Geometry: final body of the model. Coordinates: model frame, mm. Face numbers are marked on the shaded views. A direction names the side the tool comes from. Coordinates: 2 decimals unless noted, no trailing zeros. Loops run counter-clockwise (first coordinate to the right, second up) from the corner with the lowest first, then second, coordinate; pieces in that order, holes last. Notation, with made-up numbers: (5.5, 20.5) - (25.5, 20.5) arc R24 ccw to (25.5, 51.5) - close; hole circle Ø11 at (12, 54.25). An arc over 180 degrees is marked (long way). Put each result on its own line as item: value. Start each with the question number.
1) Material intervals for line 1 along X through (y, z) = (2.2, 0); line 2 along X through (y, z) = (9.5, 0); line 3 along Y through (x, z) = (-10.5, -5), sorted ascending. Write a range as from..to.
2) Section C-C on x = 5. Output: boundary loops of the cut face in (y, z), and give its area (3 significant figures).
3) Contact query for flat-ended pins moving along their axis: pin 1 Ø6 at (x, z) = (-10, 0) entering from -Y; pin 2 Ø1.5 at (x, z) = (-3, -2) entering from +Y; pin 3 Ø1 at (x, y) = (12.5, 10.5) entering from -Z. Output: stop coordinate, or through.
4) Reachability of the marked faces 3, 4 and 5 from +Z, -Z, +X, -X, +Y, -Y: full face, straight path, thin tool, end or side. Return the list, or none.
5) Section B-B on x = 8.5. Output: boundary loops of the cut face in (y, z).
6) Draft query along X for the marked faces 1 and 2. Return one class per face: +X half, -X half, draft (parallel to the pull), parting line (faces both ways), or undercut.
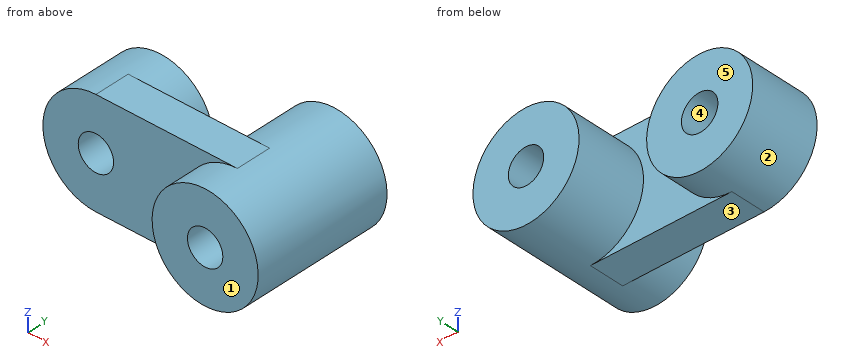
```python
from build123d import *

# Parameters (mm, degrees)
CROQUIS1_R                   = 2.5
SALIENTE_EXTRUIR1_DEPTH      = 5
CROQUIS2_R                   = 7.5
CROQUIS2_R_2                 = 2.58081611
SALIENTE_EXTRUIR2_DEPTH      = 5
SALIENTE_EXTRUIR3_DEPTH      = 10
SALIENTE_EXTRUIR3_DEPTH_BACK = 10
CROQUIS3_R                   = 7.5
CROQUIS3_R_2                 = 2.5


with BuildPart() as part:
    # Croquis1 → Saliente-Extruir1 (new body)
    with BuildSketch(Plane(origin=(0, 0, 0), x_dir=(1, 0, 0), z_dir=(0, 1, 0))):
        with BuildLine():
            ThreePointArc((-10, 7.5), (-17.5, 0), (-10, -7.5))
            Line((-10, -7.5), (10, -7.5))
            ThreePointArc((10, -7.5), (17.5, 0), (10, 7.5))
            Line((10, 7.5), (-10, 7.5))
        make_face()
        with Locations(Location((-10, 0, 0), (0, 0, 270))):
            Circle(CROQUIS1_R, mode=Mode.SUBTRACT)
        with Locations(Location((10, 0, 0), (0, 0, 270))):
            Circle(CROQUIS1_R, mode=Mode.SUBTRACT)
    extrude(amount=SALIENTE_EXTRUIR1_DEPTH)

    # Croquis2 → Saliente-Extruir2 (add)
    with BuildSketch(Plane(origin=(0, 5, 0), x_dir=(1, 0, 0), z_dir=(0, 1, 0))):
        with Locations(Location((-10, 0, 0), (0, 0, 270))):
            Circle(CROQUIS2_R)
        with Locations(Location((-10, 0, 0), (0, 0, 270))):
            Circle(CROQUIS2_R_2, mode=Mode.SUBTRACT)
    extrude(amount=SALIENTE_EXTRUIR2_DEPTH)

    # Croquis3 → Saliente-Extruir3 (add, two sides: drawn at the far end of the back side and taken through both)
    with BuildSketch(Plane(origin=(0, 5, 0), x_dir=(1, 0, 0), z_dir=(0, 1, 0)).offset(-SALIENTE_EXTRUIR3_DEPTH_BACK)):
        with Locations(Location((10, 0, 0), (0, 0, 270))):
            Circle(CROQUIS3_R)
        with Locations(Location((10, 0, 0), (0, 0, 270))):
            Circle(CROQUIS3_R_2, mode=Mode.SUBTRACT)
    extrude(amount=SALIENTE_EXTRUIR3_DEPTH + SALIENTE_EXTRUIR3_DEPTH_BACK)


solid = part.part
```
Answer block:
1. line 1: x = -17.5..-12.5, -7.5..7.5, 12.5..17.5
1. line 2: x = -17.5..-12.58, -7.42..-2.5, 2.5..7.5, 12.5..17.5
1. line 3: y = 0..10
2. outline: (-5, -5.59) - (0, -5.59) - (0, -7.5) - (5, -7.5) - (5, -5.59) - (15, -5.59) - (15, 5.59) - (5, 5.59) - (5, 7.5) - (0, 7.5) - (0, 5.59) - (-5, 5.59) - close
2. area: 243 mm²
3. pin 1: stops at y = 0
3. pin 2: stops at y = 10
3. pin 3: stops at z = -7.23
4. face 3: -Z, +X, -X, +Y, -Y
4. face 4: +Y
4. face 5: +Z, -Z, -X, +Y
5. outline: (-5, -7.35) - (0, -7.35) - (0, -7.5) - (5, -7.5) - (5, -7.35) - (15, -7.35) - (15, -2) - (-5, -2) - close; (-5, 2) - (15, 2) - (15, 7.35) - (5, 7.35) - (5, 7.5) - (0, 7.5) - (0, 7.35) - (-5, 7.35) - close
6. face 1: draft
6. face 2: undercut
